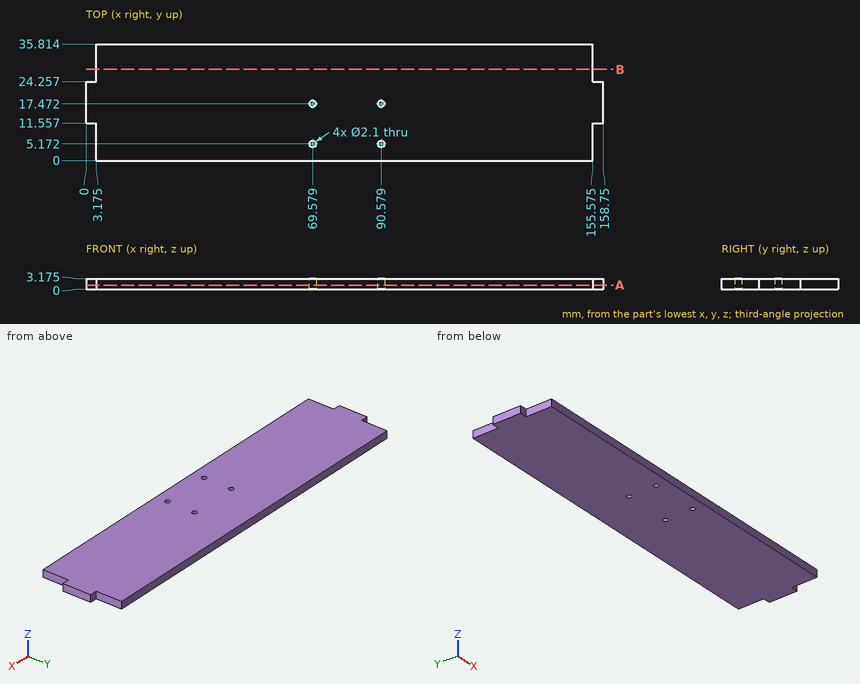
Drawing for the job (mm, zero at the part's lowest x, y, z). Round coordinates to 2 decimals unless told otherwise and drop trailing zeros. Order: outer loops, then holes, each group sorted by start corner. A loop starts at its lowest first (then second) coordinate and runs counter-clockwise, first axis right, second up. Notation, with made-up numbers: (74, -28.5) -> (101, -28.5) arc R15 cw to (101, -15.5) -> close; hole circle Ø4 at (6, 24). An arc over 180 degrees is marked (long way). Put each result on its own line as item: value.
Q1. Band-saw the part on A-A (z = 1.2). State how many separate pieces and enclosed holes the cut face has, and give its area (4 significant figures).
From the geometry:
separate pieces: 1
enclosed holes: 4
area: 5,525 mm2
Q2. Band-saw the part on B-B (y = 28). Give the cut face in (x, z) (3 decimals), and give its area (3 significant figures).
From the geometry:
outline: (3.175, 0) -> (155.575, 0) -> (155.575, 3.175) -> (3.175, 3.175) -> close
area: 484 mm2
Q3. Pin check, flat tips, straight feed: pin 1 Ø1.3 at (x, y) = (69.58, 5.17) entering from -Z; pin 2 Ø1 at (x, z) = (1.5, 1.5) entering from -Y; pin 3 Ø1.6 at (y, z) = (29.5, 1.5) entering from -X (3 decimals); pin 4 Ø1.6 at (y, z) = (32.5, 2) entering from +X (3 decimals). Stop position of each tip, or through.
From the geometry:
pin 1: passes through
pin 2: stops at y = 11.56
pin 3: stops at x = 3.175
pin 4: stops at x = 155.575
Q4. Wall check: line 1 (X direction, y = 2.5, z = 0.8) (3 decimals). Give the ranges that are in metal, low to high. Write a range as [from, to].
From the geometry:
line 1: x = [3.175, 155.575]
